```python
from build123d import *

# Parameters (mm, degrees)
SKETCH1_R           = 5
BOSS_EXTRUDE1_DEPTH = 10
FILLET1_R           = 5


with BuildPart() as part:
    # Sketch1 → Boss-Extrude1 (new body)
    with BuildSketch(Plane(origin=(0, 0, 0), x_dir=(1, 0, 0), z_dir=(0, 1, 0))):
        with BuildLine():
            Line((-2.083872426, 47.950209336), (-2.083872426, 34.937908863))
            ThreePointArc((-2.083872426, 34.937908863), (-24.748737342, 24.748737342), (-34.937908863, 2.083872426))
            Line((-34.937908863, 2.083872426), (-47.950209336, 2.083872426))
            Line((-47.950209336, 2.083872426), (-47.950209336, 8.976599642))
            Line((-47.950209336, 8.976599642), (-53.642672207, 8.976599642))
            Line((-53.642672207, 8.976599642), (-53.642672207, -8.976599642))
            Line((-53.642672207, -8.976599642), (-47.950209336, -8.976599642))
            Line((-47.950209336, -8.976599642), (-47.950209336, -2.083872426))
            Line((-47.950209336, -2.083872426), (-34.937908863, -2.083872426))
            ThreePointArc((-34.937908863, -2.083872426), (-24.748737342, -24.748737342), (-2.083872426, -34.937908863))
            Line((-2.083872426, -34.937908863), (-2.083872426, -47.950209336))
            Line((-2.083872426, -47.950209336), (-8.976599642, -47.950209336))
            Line((-8.976599642, -47.950209336), (-8.976599642, -53.642672207))
            Line((-8.976599642, -53.642672207), (8.976599642, -53.642672207))
            Line((8.976599642, -53.642672207), (8.976599642, -47.950209336))
            Line((8.976599642, -47.950209336), (2.083872426, -47.950209336))
            Line((2.083872426, -47.950209336), (2.083872426, -34.937908863))
            ThreePointArc((2.083872426, -34.937908863), (24.748737342, -24.748737342), (34.937908863, -2.083872426))
            Line((34.937908863, -2.083872426), (47.950209336, -2.083872426))
            Line((47.950209336, -2.083872426), (47.950209336, -8.976599642))
            Line((47.950209336, -8.976599642), (53.642672207, -8.976599642))
            Line((53.642672207, -8.976599642), (53.642672207, 8.976599642))
            Line((53.642672207, 8.976599642), (47.950209336, 8.976599642))
            Line((47.950209336, 8.976599642), (47.950209336, 2.083872426))
            Line((47.950209336, 2.083872426), (34.937908863, 2.083872426))
            ThreePointArc((34.937908863, 2.083872426), (24.748737342, 24.748737342), (2.083872426, 34.937908863))
            Line((2.083872426, 34.937908863), (2.083872426, 47.950209336))
            Line((2.083872426, 47.950209336), (8.976599642, 47.950209336))
            Line((8.976599642, 47.950209336), (8.976599642, 53.642672207))
            Line((8.976599642, 53.642672207), (-8.976599642, 53.642672207))
            Line((-8.976599642, 53.642672207), (-8.976599642, 47.950209336))
            Line((-8.976599642, 47.950209336), (-2.083872426, 47.950209336))
        make_face()
        Circle(SKETCH1_R, mode=Mode.SUBTRACT)
    extrude(amount=BOSS_EXTRUDE1_DEPTH)

    # Fillet1
    fillet1_edges = [part.edges().sort_by_distance(p)[0] for p in [
        (2.083872426, 5, 47.950209336),
        (-2.083872426, 5, 47.950209336),
        (-47.950209336, 5, 2.083872426),
        (-47.950209336, 5, -2.083872426),
        (-2.083872426, 5, -47.950209336),
        (2.083872426, 5, -47.950209336),
        (47.950209336, 5, -2.083872426),
        (47.950209336, 5, 2.083872426),
    ]]
    fillet(fillet1_edges, radius=FILLET1_R)


solid = part.part
```
Design review of the part built by this model. Coordinates are the model's own, in mm. A direction names the side the tool comes from. Coordinates: 2 decimals unless noted, no trailing zeros. Loops run counter-clockwise (first coordinate to the right, second up) from the corner with the lowest first, then second, coordinate; pieces in that order, holes last.
Q1. We need section D-D on x = -30. State the section outline as (y, z) points, and give its area (3 significant figures).
Reported:
outline: (0, -18.03) - (10, -18.03) - (10, 18.03) - (0, 18.03) - close
area: 361 mm2
Q2. To check wall thickness, follow line 1 (Z direction, x = 0, y = 2.75); line 2 (X direction, y = 2, z = 4). State the ranges of each line that lie inside material, in increasing order.
Reported:
line 1: z = -53.64 to -5, 5 to 53.64
line 2: x = -53.64 to -46.89, -34.77 to -3, 3 to 34.77, 46.89 to 53.64
Q3. We need section B-B on z = 0. State the section outline as (x, y) points.
Reported:
outline: (-53.64, 0) - (-5, 0) - (-5, 10) - (-53.64, 10) - close; (5, 0) - (53.64, 0) - (53.64, 10) - (5, 10) - close
Q4. We need section A-A on x = 0. State the section outline as (y, z) points, and give its area (3 significant figures).
Reported:
outline: (0, -53.64) - (10, -53.64) - (10, -5) - (0, -5) - close; (0, 5) - (10, 5) - (10, 53.64) - (0, 53.64) - close
area: 973 mm2
Q5. For pin 1 (4 mm diameter, centred on x = -37, y = 5, fed in from +Z); pin 2 (9 mm diameter, centred on x = 0, z = 0, fed in from -Y); pin 3 (4 mm diameter, centred on y = 7, z = -14.5, fed in from +X); pin 4 (3 mm diameter, centred on y = 7.5, z = -29.5, fed in from -X), all flat-tipped, find the tip position at first contact; note any pin that passes through.
Reported:
pin 1: stops at z = 2.08
pin 2: passes through
pin 3: stops at x = 32.69
pin 4: stops at x = -21
Q6. The part is to be moulded in two halves that separate along X. For faces 5 (the face through (53.643, 5, 0)), 6 (the face through (-3.51, 5.07, -46.447)), 7 (the face through (46.447, 5.07, -3.51)), say which applies: +X half, -X half, draft (parallel to the pull), parting line (faces both ways), or undercut.
Reported:
face 5: +X half
face 6: -X half
face 7: undercut
Q7. Tool access review of faces 1 (the face through (51, 5, 8.977)), 2 (the face through (3.587, 5.07, -46.524)), 3 (the face through (-51, 5, -8.977)), 4 (the face through (-3.51, 5.07, 46.447)): name each direction out of +Z, -Z, +X, -X, +Y, -Y from which nothing blocks a thin tool from reaching the whole face with its end or side.
Reported:
face 1: +Z, +X, +Y, -Y
face 2: +X, +Y, -Y
face 3: -Z, -X, +Y, -Y
face 4: -X, +Y, -Y
Q8. We need section C-C on z = 37.5. State the section outline as (x, y) points.
Reported:
outline: (-2.08, 0) - (2.08, 0) - (2.08, 10) - (-2.08, 10) - close
